Design review of the part built by this model. Coordinates are the model's own, in mm. Face numbers are marked on the shaded views. A direction names the side the tool comes from. Coordinates: 2 decimals unless noted, no trailing zeros. Loops run counter-clockwise (first coordinate to the right, second up) from the corner with the lowest first, then second, coordinate; pieces in that order, holes last. Notation, with made-up numbers: (73.5, 43.5) - (125.5, 43.5) arc R21 cw to (125.5, 67.5) - close; hole circle Ø2 at (50, -26). An arc over 180 degrees is marked (long way). One line per question, with ' | ' between items.
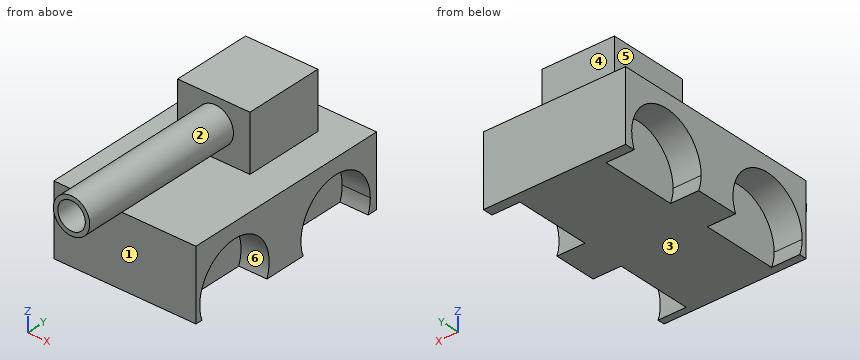
from build123d import *

# Parameters (mm, degrees)
F0_W      = 64.230248332
F0_H      = 95.7897491753
F1_DEPTH  = 31.75
F4_DEPTH  = 12.7
F5_DEPTH  = 12.7
F6_W      = 32.6707493514
F6_H      = 36.0044999979
F7_DEPTH  = 25.4
F8_R      = 8.2239975994
F9_DEPTH  = 76.2
F10_R     = 6.2290995739
F11_DEPTH = 76.2


with BuildPart() as f1:
    # F0 (on Top) → F1 (new body)
    with BuildSketch(Plane.XY):
        with Locations((-0.8889995515, -2.6670005172)):
            Rectangle(F0_W, F0_H)
    extrude(amount=F1_DEPTH)

    # F2 (on face) → F4 (cut)
    with BuildSketch(Plane.YZ.offset(31.2261246145)):
        with BuildLine():
            Line((-47.3948020572, 0), (-12.907678998, 0))
            ThreePointArc((-12.907678998, 0), (-30.1512405276, 24.8333887155), (-47.3948020572, 0))
        make_face()
        with BuildLine():
            ThreePointArc((40.7211401539, 0), (41.5896545425, 3.1629956827), (41.8822641726, 6.4299879596))
            ThreePointArc((41.8822641726, 6.4299879596), (20.2309505583, 24.521699667), (6.2747455163, 0))
            Line((6.2747455163, 0), (40.7211401539, 0))
        make_face()
    extrude(amount=-F4_DEPTH, mode=Mode.SUBTRACT)

    # F3 (on face) → F5 (cut)
    with BuildSketch(Plane(origin=(-33.0041237175, 0, 0), x_dir=(0, -1, 0), z_dir=(-1, 0, 0))):
        with BuildLine():
            ThreePointArc((-6.4749563765, 0), (-5.4877667655, 3.3604332928), (-5.1546871083, 6.8469950929))
            ThreePointArc((-5.1546871083, 6.8469950929), (-27.055845807, 24.9285123344), (-40.6636116374, 0))
            Line((-40.6636116374, 0), (-6.4749563765, 0))
        make_face()
        with BuildLine():
            ThreePointArc((48.4297908844, 6.8469950929), (26.592859866, 24.8625205102), (13.0552904295, 0))
            Line((13.0552904295, 0), (47.1045045567, 0))
            ThreePointArc((47.1045045567, 0), (48.0954229104, 3.3599574658), (48.4297908844, 6.8469950929))
        make_face()
    extrude(amount=-F5_DEPTH, mode=Mode.SUBTRACT)

    # F6 (on face) → F7 (join)
    with BuildSketch(Plane.XY.offset(31.75)):
        with Locations((-0.6667496637, 14.3351249862)):
            Rectangle(F6_W, F6_H)
    extrude(amount=F7_DEPTH)

    # F8 (on face) → F9 (join)
    with BuildSketch(Plane.XZ.offset(3.6671250127)):
        with Locations((0, 45.4501248896)):
            Circle(F8_R)
    extrude(amount=F9_DEPTH)

    # F10 (on face) → F11 (cut)
    with BuildSketch(Plane.XZ.offset(79.8671250127)):
        with Locations((0, 45.4501248896)):
            Circle(F10_R)
    extrude(amount=-F11_DEPTH, mode=Mode.SUBTRACT)


solid = f1.part
Q1. Take a section at B-B (x = -13). Give the boundary of the cut face in (y, z), plus the area to 3 significant figures.
Returned:
outline: (-50.56, 0) - (45.23, 0) - (45.23, 31.75) - (32.34, 31.75) - (32.34, 57.15) - (-3.67, 57.15) - (-3.67, 31.75) - (-50.56, 31.75) - close | area: 3,960 mm²
Q2. Take a section at D-D (x = 0). Give the boundary of the cut face in (y, z), plus the area to 3 significant figures.
Returned:
outline: (-79.87, 37.23) - (-3.67, 37.23) - (-3.67, 31.75) - (-50.56, 31.75) - (-50.56, 0) - (45.23, 0) - (45.23, 31.75) - (32.34, 31.75) - (32.34, 57.15) - (-3.67, 57.15) - (-3.67, 53.67) - (-79.87, 53.67) - (-79.87, 51.68) - (-3.67, 51.68) - (-3.67, 39.22) - (-79.87, 39.22) - close | area: 4,260 mm²
Q3. To check wall thickness, follow line 1 along Y through (x, z) = (-29, 7.5); line 2 along Z through (x, y) = (0, -32); line 3 along Y through (x, z) = (27, 20.5). State the ranges of each line that lie inside material, in increasing order.
Returned:
line 1: y = -50.56 to -48.42, -11.74 to 5.17, 41.97 to 45.23 | line 2: z = 0 to 31.75, 37.23 to 39.22, 51.68 to 53.67 | line 3: y = -50.56 to -42.01, -18.29 to 11.67, 35.33 to 45.23
Q4. For pin 1 (7.5 mm diameter, centred on y = 19.5, z = 45.5, fed in from -X); pin 2 (16 mm diameter, centred on x = 0, z = 45.45, fed in from +Y); pin 3 (6 mm diameter, centred on x = 3.5, z = 20.5, fed in from -Y), all flat-tipped, find the tip position at first contact; note any pin that passes through.
Returned:
pin 1: stops at x = -17 | pin 2: stops at y = 32.34 | pin 3: stops at y = -50.56
Q5. Take a section at C-C (y = 3.5). Give the boundary of the cut face in (x, z).
Returned:
outline: (-33, 0) - (31.23, 0) - (31.23, 31.75) - (15.67, 31.75) - (15.67, 57.15) - (-17, 57.15) - (-17, 31.75) - (-33, 31.75) - close
Q6. Take a section at A-A (y = -41.5). Give the boundary of the cut face in (x, z).
Returned:
outline: (-33, 21.21) - (-20.3, 21.21) - (-20.3, 0) - (18.53, 0) - (18.53, 20.92) - (31.23, 20.92) - (31.23, 31.75) - (-33, 31.75) - close; circle Ø16.45 at (0, 45.45); hole circle Ø12.46 at (0, 45.45)
Q7. Tool access review of the marked faces 4, 5 and 6: name each direction out of +Z, -Z, +X, -X, +Y, -Y from which nothing blocks a thin tool from reaching the whole face with its end or side.
Returned:
face 4: +Z, +X, -X, +Y | face 5: +Z, -X, +Y, -Y | face 6: +X
Q8. Draft analysis for pull direction Z (two halves, no side actions). For the marked faces 1, 2 and 3, state which applies: +Z half, -Z half, draft (parallel to the pull), parting line (faces both ways), or undercut.
Returned:
face 1: draft | face 2: undercut | face 3: -Z half
